Could you check a few things on this model? Use its own coordinates, in mm. Face numbers are marked on the shaded views. A direction names the side the tool comes from. Give positions to 0.01 mm unless a question says otherwise; leave off trailing zeros. Write each loop counter-clockwise with the first axis right and the second up, starting at its lowest first coordinate (ties: lowest second). Pieces come first, ordered by that corner, then holes. Notation, with made-up numbers: (9.25, -18.5) - (68.25, -18.5) arc R23 cw to (68.25, 15.5) - close; hole circle Ø2 at (-28, 64.25). An arc over 180 degrees is marked (long way). Write item = value, one per line.
from build123d import *

# Parameters (mm, degrees)
TUBO_CUADRADO_40_X_40_X_4_1_DEPTH = 40
EXTRUDE1_REACH                    = 62


with BuildPart() as part:
    # Sketch6 → Tubo cuadrado 40 X 40 X 4(1) (new body)
    with BuildSketch(Plane(origin=(0, 0, 0), x_dir=(0, 0, -1), z_dir=(1, 0, 0))):
        with BuildLine():
            Line((-12, -20), (12, -20))
            ThreePointArc((12, -20), (17.656854249, -17.656854249), (20, -12))
            Line((20, -12), (20, 12))
            ThreePointArc((20, 12), (17.656854249, 17.656854249), (12, 20))
            Line((12, 20), (-12, 20))
            ThreePointArc((-12, 20), (-17.656854249, 17.656854249), (-20, 12))
            Line((-20, 12), (-20, -12))
            ThreePointArc((-20, -12), (-17.656854249, -17.656854249), (-12, -20))
        make_face()
        with BuildLine():
            Line((-12, -16), (12, -16))
            ThreePointArc((12, -16), (14.828427125, -14.828427125), (16, -12))
            Line((16, -12), (16, 12))
            ThreePointArc((16, 12), (14.828427125, 14.828427125), (12, 16))
            Line((12, 16), (-12, 16))
            ThreePointArc((-12, 16), (-14.828427125, 14.828427125), (-16, 12))
            Line((-16, 12), (-16, -12))
            ThreePointArc((-16, -12), (-14.828427125, -14.828427125), (-12, -16))
        make_face(mode=Mode.SUBTRACT)
    extrude(amount=TUBO_CUADRADO_40_X_40_X_4_1_DEPTH)

    # Sketch2 → Extrude1 (cut, up to next)
    with BuildSketch(Plane.XY.offset(20), mode=Mode.PRIVATE) as extrude1_sk1:
        Polygon((-9.656854249, 24), (44, -29.656854249), (44, 24), align=None)
    extrude1_tool1 = extrude(extrude1_sk1.sketch, amount=-EXTRUDE1_REACH, mode=Mode.PRIVATE) & part.part
    add(extrude1_tool1.solids().sort_by_distance((26.114382, 6.114382, 20))[0], mode=Mode.SUBTRACT)


solid = part.part
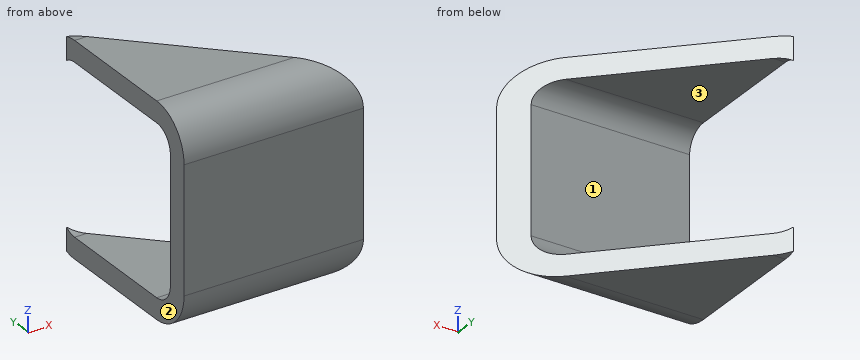
1. If we section it at A-A, the plane y = -10: Please give me the cut outline in (x, z).
Filled sheet:
outline = (0, -20) - (24.34, -20) - (24.34, -16) - (0, -16) - close; (0, 16) - (24.34, 16) - (24.34, 20) - (0, 20) - close
2. If we section it at B-B, the plane x = 17.5: Please give me the cut outline in (y, z).
Filled sheet:
outline = (-20, -12) arc R8 ccw to (-12, -20) - (-3.16, -20) - (-3.16, -16) - (-12, -16) arc R4 cw to (-16, -12) - (-16, 12) arc R4 cw to (-12, 16) - (-3.16, 16) - (-3.16, 20) - (-12, 20) arc R8 ccw to (-20, 12) - close
3. If we section it at C-C, the plane y = 9: Please give me the cut outline in (x, z).
Filled sheet:
outline = (0, -20) - (5.34, -20) - (5.34, -16) - (0, -16) - close; (0, 16) - (5.34, 16) - (5.34, 20) - (0, 20) - close
4. I need wall thicknesses on line 1 (Z direction, x = 3.5, y = 3); line 2 (Y direction, x = 6.5, z = 9.5); line 3 (Y direction, x = 24, z = 15). Which ranges of each line are inside material? Lowest first, please.
Filled sheet:
line_1 = -20 to -16, 16 to 20
line_2 = -20 to -16
line_3 = -19.42 to -14.65
5. Which directions (+Z, -Z, +X, -X, +Y, -Y) give clear straight access to the entire face, cutting with the end or side of a thin tool? Please do the marked faces 1, 2 and 3.
Filled sheet:
face_1 = +X, -X, +Y
face_2 = +Z, -Z, -X, +Y, -Y
face_3 = +X, -X
6. For pin 1 (4 mm diameter, centred on x = 19, z = 6, fed in from +Y), with a flat end and sliding along its axis, tell me the tip position at first contact or that it passes through.
Filled sheet:
pin_1 = -16
7. If we section it at D-D, the plane z = -0.5: Please give me the cut outline in (x, y).
Filled sheet:
outline = (0, -20) - (34.34, -20) - (30.34, -16) - (0, -16) - close
